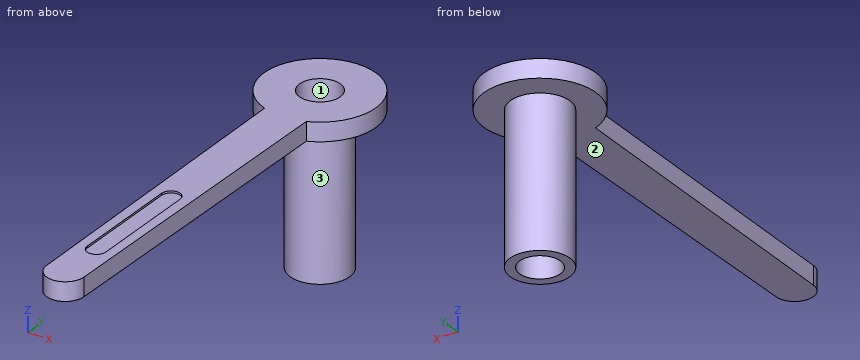
```python
from build123d import *

# Parameters (mm, degrees)
PAD_DEPTH    = 1
POCKET_DEPTH = 0.1


with BuildPart() as part:
    # Sketch → Revolution (revolve)
    with BuildSketch(Plane.YZ):
        Polygon((-3, 0), (-1.1, 0), (-1.1, -9), (-1.6, -9), (-1.6, -1), (-3, -1), align=None)
    revolve(axis=Axis((0, 0, 0), (0, 0, 1)))

    # Sketch001 (on Face1 of Revolution) → Pad (new body)
    with BuildSketch(Plane(origin=(0, 0, 0), x_dir=(0, -1, 0), z_dir=(0, 0, 1))):
        with BuildLine():
            Line((2.781074, 1.125), (2.781074, -1.125))
            Line((2.781074, -1.125), (20.507022, -1))
            ThreePointArc((20.507022, -1), (21.5, 0), (20.507022, 1))
            Line((2.781074, 1.125), (20.507022, 1))
        make_face()
    extrude(amount=-PAD_DEPTH)

    # Sketch002 (on Face2 of Pad) → Pocket (cut)
    with BuildSketch(Plane(origin=(0, 0, 0), x_dir=(0, -1, 0), z_dir=(0, 0, 1))):
        with BuildLine():
            ThreePointArc((12, 0.5), (11.5, 0), (12, -0.5))
            Line((12, -0.5), (18, -0.5))
            ThreePointArc((18, -0.5), (18.5, 0), (18, 0.5))
            Line((12, 0.5), (18, 0.5))
        make_face()
    extrude(amount=-POCKET_DEPTH, mode=Mode.SUBTRACT)


solid = part.part
```
Verification items for the finished model (mm, model axes). Face numbers are marked on the shaded views. Coordinates: 2 decimals unless noted, no trailing zeros. Order: outer loops, then holes, each group sorted by start corner. A loop starts at its lowest first (then second) coordinate and runs counter-clockwise, first axis right, second up. Notation, with made-up numbers: (12, -30) - (26, -30) arc R17 ccw to (26, 2) - close; hole circle Ø1 at (11, 9). An arc over 180 degrees is marked (long way). Return JSON: item names as keys, results as strings.
(1) Section check D-D, the plane y = -11.75. Record the cut outline in (x, z).
Filled sheet:
{"outline": "(-1.06, -1) - (1.06, -1) - (1.06, 0) - (0.43, 0) - (0.43, -0.1) - (-0.43, -0.1) - (-0.43, 0) - (-1.06, 0) - close"}
(2) Section check C-C, the plane y = -16.5. Record the cut outline in (x, z), and give its area (3 significant figures).
Filled sheet:
{"outline": "(-1.03, -1) - (1.03, -1) - (1.03, 0) - (0.5, 0) - (0.5, -0.1) - (-0.5, -0.1) - (-0.5, 0) - (-1.03, 0) - close", "area": "1.96 mm^2"}
(3) Mould release check, pull along X, two halves, no side actions. Record for the marked faces 1, 2 and 3: pulls with the +X half, pulls with the -X half, needs draft (parallel to the pull), parting line crosses it, or undercut.
Filled sheet:
{"face 1": "undercut", "face 2": "needs draft", "face 3": "parting line crosses it"}
(4) Thickness scan on line 1 along X through (y, z) = (0, -2.5); line 2 along Z through (x, y) = (-0.05, -18); line 3 along Y through (x, z) = (-0.25, -0.25). Record the ranges inside material, lowest first.
Filled sheet:
{"line 1": "x = -1.6 to -1.1, 1.1 to 1.6", "line 2": "z = -1 to -0.1", "line 3": "y = -21.47 to -1.07, 1.07 to 2.99"}
(5) Section check B-B, the plane z = -1.25. Record the cut outline in (x, y).
Filled sheet:
{"outline": "circle Ø3.2 at (0, 0); hole circle Ø2.2 at (0, 0)"}
(6) Go/stop test with flat-tipped pins: pin 1 (1 mm diameter, centred on x = 0.5, z = -2, fed in from +Y); pin 2 (1.8 mm diameter, centred on x = 1, y = -9.5, fed in from -Z); pin 3 (1.5 mm diameter, centred on y = -1, z = -3, fed in from +X). Record where each tip stops, or that it passes through.
Filled sheet:
{"pin 1": "stops at y = 1.6", "pin 2": "stops at z = -1", "pin 3": "stops at x = 1.58"}
(7) Section check A-A, the plane y = 0. Record the cut outline in (x, z), and give its area (3 significant figures).
Filled sheet:
{"outline": "(-3, -1) - (-1.6, -1) - (-1.6, -9) - (-1.1, -9) - (-1.1, 0) - (-3, 0) - close; (1.1, -9) - (1.6, -9) - (1.6, -1) - (3, -1) - (3, 0) - (1.1, 0) - close", "area": "11.8 mm^2"}
